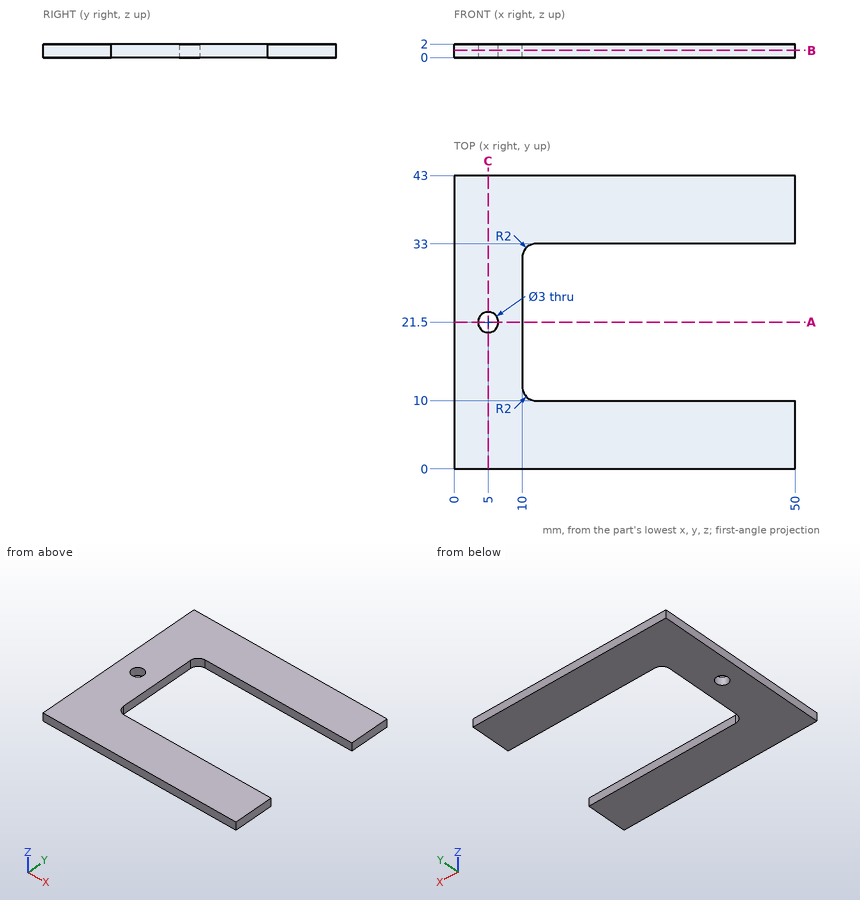
Geometry: see drawing. Coordinates: mm, zero at the bounding-box minimum. Coordinates: 2 decimals unless noted, no trailing zeros. Write each loop counter-clockwise with the first axis right and the second up, starting at its lowest first coordinate (ties: lowest second). Pieces come first, ordered by that corner, then holes. Notation, with made-up numbers: (59.5, 74.5) - (94.5, 74.5) arc R31 ccw to (94.5, 98.5) - close; hole circle Ø6 at (77, -39). An arc over 180 degrees is marked (long way). Put each result on its own line as item: value. Start each with the question number.
1) Ray query, L1, parallel to Y at x = 36, z = 1.6; L2, parallel to Y at x = 5, z = 1.65; L3, parallel to X at y = 16, z = 1.75. Return the intervals inside material, ascending.
2) Cut plane C-C (x = 5). Return the cut outline in (y, z), plus the area to 3 significant figures.
3) Contact query for a flat-ended pin moving along its axis: pin 1 (1 mm diameter, centred on x = 6, z = 1, fed in from -Y). Output: stop coordinate, or through.
4) Cut plane B-B (z = 1.05). Return the cut outline in (x, y).
5) Cut plane A-A (y = 21.5). Return the cut outline in (x, z).
Resolved:
1. L1: y = 0 to 10, 33 to 43
1. L2: y = 0 to 20, 23 to 43
1. L3: x = 0 to 10
2. outline: (0, 0) - (20, 0) - (20, 2) - (0, 2) - close; (23, 0) - (43, 0) - (43, 2) - (23, 2) - close
2. area: 80.0 mm2
3. pin 1: stops at y = 0
4. outline: (0, 0) - (50, 0) - (50, 10) - (12, 10) arc R2 cw to (10, 12) - (10, 31) arc R2 cw to (12, 33) - (50, 33) - (50, 43) - (0, 43) - close; hole circle Ø3 at (5, 21.5)
5. outline: (0, 0) - (3.5, 0) - (3.5, 2) - (0, 2) - close; (6.5, 0) - (10, 0) - (10, 2) - (6.5, 2) - close
